Read the model definition and answer for the solid it produces. Units are mm, in the model's axes. Face numbers are marked on the shaded views. Round coordinates to 2 decimals unless told otherwise and drop trailing zeros. Write each loop counter-clockwise with the first axis right and the second up, starting at its lowest first coordinate (ties: lowest second). Pieces come first, ordered by that corner, then holes. Notation, with made-up numbers: (-0.5, 10) -> (24.5, 10) arc R8 ccw to (24.5, 18) -> close; hole circle Ø9 at (-11, 14). An arc over 180 degrees is marked (long way). Return JSON: item names as keys, results as strings. Group by question number.
(1) Given pin 1 (3.5 mm diameter, centred on x = 0, y = -11, fed in from +Z); pin 2 (1 mm diameter, centred on y = 13, z = 11.5, fed in from +X); pin 3 (4 mm diameter, centred on y = 13, z = 11, fed in from -X); pin 4 (3 mm diameter, centred on x = 7.78, y = -7.78, fed in from -Z), each flat-ended and moving along its own axis, determine where each tip first touches the part or whether it passes through.
(2) The mould has two halves that part along Y. Classify the marked faces 1 and 2: released by +Y, released by -Y, zero draft, split by the parting line, or undercut.
(3) A cutting plane is placed at A-A on z = 57.5. Give the vertices of the cut face in (x, y), then the cut area to 3 significant figures.
(4) Straight lines are drawn through the part: line 1 (Z direction, x = 9.25, y = 6.5); line 2 (Y direction, x = 11, z = 2.5); line 3 (Y direction, x = 2.25, z = 24). For each, find the intervals that lie inside material, in ascending order.
```python
from build123d import *

# Parameters (mm, degrees)
SALIENTE_EXTRUIR1_DEPTH = 60
CROQUIS2_R              = 1.6
CORTAR_EXTRUIR1_DEPTH   = 20
CORTAR_EXTRUIR2_START   = -10
CORTAR_EXTRUIR2_DEPTH   = 3.5
CROQUIS4_R              = 4.1
CORTAR_EXTRUIR3_DEPTH   = 122.86057607


with BuildPart() as part:
    # Croquis1 → Saliente-Extruir1 (new body)
    with BuildSketch(Plane.XY):
        Polygon((15, -6.213203436), (15, 6.213203436), (6.213203436, 15), (-6.213203436, 15), (-15, 6.213203436), (-15, -6.213203436), (-6.213203436, -15), (6.213203436, -15), align=None)
    saliente_extruir1 = extrude(amount=SALIENTE_EXTRUIR1_DEPTH)

    # Croquis2 → Cortar-Extruir1 (cut)
    with BuildSketch(Plane(origin=(0, 0, 0), x_dir=(-1, 0, 0), z_dir=(0, 0, -1))):
        with Locations((0, 11)):
            Circle(CROQUIS2_R)
        with Locations((7.778174593, 7.778174593)):
            Circle(CROQUIS2_R)
        with Locations((11, 0)):
            Circle(CROQUIS2_R)
        with Locations((7.778174593, -7.778174593)):
            Circle(CROQUIS2_R)
        with Locations((0, -11)):
            Circle(CROQUIS2_R)
        with Locations((-7.778174593, -7.778174593)):
            Circle(CROQUIS2_R)
        with Locations((-11, 0)):
            Circle(CROQUIS2_R)
        with Locations((-7.778174593, 7.778174593)):
            Circle(CROQUIS2_R)
    cortar_extruir1 = extrude(amount=-CORTAR_EXTRUIR1_DEPTH, mode=Mode.SUBTRACT)

    # Croquis3 → Cortar-Extruir2 (cut)
    with BuildSketch(Plane(origin=(0, 0, 0), x_dir=(-1, 0, 0), z_dir=(0, 0, -1)).offset(CORTAR_EXTRUIR2_START)):
        Polygon((-2.75, 12.58771324), (-2.75, 18.463203436), (2.75, 23.963203436), (2.75, 12.58771324), (2.75, 9.41228676), (0, 7.824573519), (-2.75, 9.41228676), align=None)
        Polygon((6.956313744, 10.84540104), (11.110912703, 15), (18.889087297, 15), (10.84540104, 6.956313744), (8.600035443, 4.710948146), (5.532808996, 5.532808996), (4.710948146, 8.600035443), align=None)
        Polygon((12.58771324, 2.75), (18.463203436, 2.75), (23.963203436, -2.75), (12.58771324, -2.75), (9.41228676, -2.75), (7.824573519, 0), (9.41228676, 2.75), align=None)
        Polygon((10.84540104, -6.956313744), (15, -11.110912703), (15, -18.889087297), (6.956313744, -10.84540104), (4.710948146, -8.600035443), (5.532808996, -5.532808996), (8.600035443, -4.710948146), align=None)
        Polygon((2.75, -12.58771324), (2.75, -18.463203436), (-2.75, -23.963203436), (-2.75, -12.58771324), (-2.75, -9.41228676), (0, -7.824573519), (2.75, -9.41228676), align=None)
        Polygon((-6.956313744, -10.84540104), (-11.110912703, -15), (-18.889087297, -15), (-10.84540104, -6.956313744), (-8.600035443, -4.710948146), (-5.532808995, -5.532808996), (-4.710948146, -8.600035443), align=None)
        Polygon((-12.58771324, -2.75), (-18.463203436, -2.75), (-23.963203436, 2.75), (-12.58771324, 2.75), (-9.41228676, 2.75), (-7.824573519, 0), (-9.41228676, -2.75), align=None)
        Polygon((-10.84540104, 6.956313744), (-15, 11.110912703), (-15, 18.889087297), (-6.956313744, 10.84540104), (-4.710948146, 8.600035443), (-5.532808996, 5.532808996), (-8.600035443, 4.710948146), align=None)
    cortar_extruir2 = extrude(amount=-CORTAR_EXTRUIR2_DEPTH, mode=Mode.SUBTRACT)

    # Simetría1: Saliente-Extruir1, Cortar-Extruir1, Cortar-Extruir2 across plane
    add(saliente_extruir1.mirror(Plane.XY.offset(60)))
    add(cortar_extruir1.mirror(Plane.XY.offset(60)), mode=Mode.SUBTRACT)
    add(cortar_extruir2.mirror(Plane.XY.offset(60)), mode=Mode.SUBTRACT)

    # Croquis4 → Cortar-Extruir3 (cut, through all)
    with BuildSketch(Plane(origin=(0, 0, 0), x_dir=(-1, 0, 0), z_dir=(0, 0, -1))):
        Circle(CROQUIS4_R)
    extrude(amount=-CORTAR_EXTRUIR3_DEPTH, mode=Mode.SUBTRACT)


solid = part.part
```
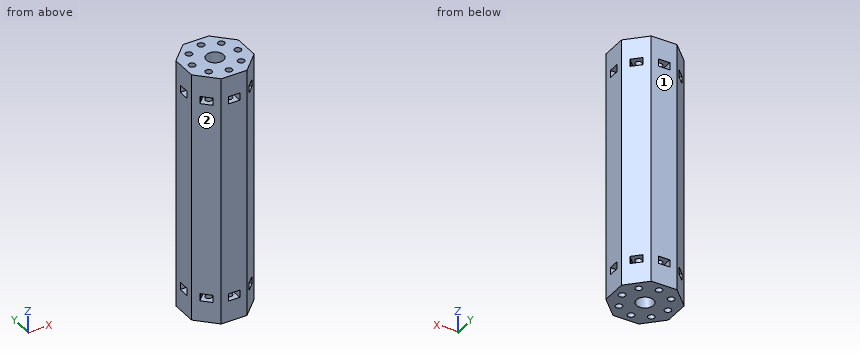
Checks:
{
 "1": {"pin 1": "stops at z = 120", "pin 2": "stops at x = 8.66", "pin 3": "stops at x = -9.95", "pin 4": "stops at z = 20"},
 "2": {"face 1": "released by +Y", "face 2": "released by -Y"},
 "3": {"outline": "(-15, -6.21) -> (-6.21, -15) -> (6.21, -15) -> (15, -6.21) -> (15, 6.21) -> (6.21, 15) -> (-6.21, 15) -> (-15, 6.21) -> close; hole circle Ø8.2 at (0, 0)", "area": "693 mm^2"},
 "4": {"line 1": "z = 0 to 10, 13.5 to 106.5, 110 to 120", "line 2": "y = -10.21 to -1.6, 1.6 to 10.21", "line 3": "y = -15 to -3.43, 3.43 to 15"}
}
